from build123d import *

# Parameters (mm, degrees)
BOSS_EXTRUDE1_DEPTH      = 1
BOSS_EXTRUDE1_DEPTH_BACK = 1
SKETCH2_R                = 30
SKETCH1_R                = 9.350852961
BOSS_EXTRUDE2_DEPTH      = 14
BOSS_EXTRUDE3_DEPTH      = 15
CIRPATTERN1_COUNT        = 3
CUT_EXTRUDE2_DEPTH       = 64.041803276
SKETCH4_R                = 1
CUT_EXTRUDE3_DEPTH       = 43
CIRPATTERN2_COUNT        = 3
CUT_EXTRUDE4_DEPTH       = 43
FILLET1_R                = 10


with BuildPart() as part:
    # Sketch2 → Boss-Extrude1 (new, two sides: drawn at the far end of the back side and taken through both)
    with BuildSketch(Plane(origin=(0, 0, 0), x_dir=(1, 0, 0), z_dir=(0, 1, 0)).offset(-BOSS_EXTRUDE1_DEPTH_BACK)):
        with Locations(Location((0, 0, 0), (0, 0, 270))):
            Circle(SKETCH2_R)
    extrude(amount=BOSS_EXTRUDE1_DEPTH + BOSS_EXTRUDE1_DEPTH_BACK)

    # Sketch1 → Boss-Extrude2 (add)
    with BuildSketch(Plane(origin=(0, 1, 0), x_dir=(1, 0, 0), z_dir=(0, 1, 0))):
        with Locations(Location((0, 0, 0), (0, 0, 90))):
            Circle(SKETCH1_R)
        Polygon((3.175426481, -5.5), (6.350852961, 0), (3.175426481, 5.5), (-3.175426481, 5.5), (-6.350852961, 0), (-3.175426481, -5.5), align=None, mode=Mode.SUBTRACT)
    extrude(amount=BOSS_EXTRUDE2_DEPTH)

    # Sketch1<3> → Boss-Extrude3 (add)
    with BuildSketch(Plane(origin=(0, 1, 0), x_dir=(1, 0, 0), z_dir=(0, 1, 0))):
        with BuildLine():
            Line((2.998219694, 26.806931157), (8.371578903, 17.5))
            Line((8.371578903, 17.5), (3.315841392, 8.74320576))
            ThreePointArc((3.315841392, 8.74320576), (4.675426481, 8.098076211), (5.913917603, 7.24320576))
            Line((5.913917603, 7.24320576), (10.969655115, 16))
            Line((10.969655115, 16), (21.716373532, 16))
            Line((21.716373532, 16), (21.716373532, 19))
            Line((21.716373532, 19), (10.969655115, 19))
            Line((10.969655115, 19), (5.596295906, 28.306931157))
            Line((5.596295906, 28.306931157), (2.998219694, 26.806931157))
        make_face()
    boss_extrude3 = extrude(amount=BOSS_EXTRUDE3_DEPTH)

    # CirPattern1: Boss-Extrude3 ×3 about axis
    cirpattern1_axis = Axis((0, 0, 0), (0, 1, 0))
    for i in range(1, CIRPATTERN1_COUNT):
        add(boss_extrude3.rotate(cirpattern1_axis, i * 360 / CIRPATTERN1_COUNT))

    # Sketch3 → Cut-Extrude2 (cut, symmetric)
    with BuildSketch(Plane(origin=(-16.454482672, 0, 9.5), x_dir=(0.5000000000000041, 0, 0.8660254037844364), z_dir=(-0.8660254037844363, 0, 0.500000000000004))):
        Polygon((-19.969655115, 2.372421116), (-21.716373532, 4.828660441), (-21.716373532, 2.372421116), align=None)
        with BuildLine():
            Line((-21.716373532, 16), (-21.716373532, 15.684973294))
            ThreePointArc((-21.716373532, 15.684973294), (-20.857104699, 15.920613096), (-19.969655115, 16))
            Line((-19.969655115, 16), (-21.716373532, 16))
        make_face()
    cut_extrude2 = extrude(amount=CUT_EXTRUDE2_DEPTH, both=True, mode=Mode.SUBTRACT)

    # Sketch4 → Cut-Extrude3 (cut)
    with BuildSketch(Plane(origin=(-16.454482672, 0, 9.5), x_dir=(0.500000000000004, 0, 0.8660254037844364), z_dir=(-0.8660254037844365, 0, 0.500000000000004))):
        with Locations((-19.969655115, 11)):
            Circle(SKETCH4_R)
    cut_extrude3 = extrude(amount=-CUT_EXTRUDE3_DEPTH, mode=Mode.SUBTRACT)

    # CirPattern2: Cut-Extrude2, Cut-Extrude3 ×3 about axis
    cirpattern2_axis = Axis((0, 1, 0), (0, 1, 0))
    add([cut_extrude2.rotate(cirpattern2_axis, i * 360 / CIRPATTERN2_COUNT) for i in range(1, CIRPATTERN2_COUNT)], mode=Mode.SUBTRACT)
    add([cut_extrude3.rotate(cirpattern2_axis, i * 360 / CIRPATTERN2_COUNT) for i in range(1, CIRPATTERN2_COUNT)], mode=Mode.SUBTRACT)

    # Sketch5 → Cut-Revolve2 (revolve, cut)
    with BuildSketch(Plane(origin=(0, 0, 0), x_dir=(0, 0, -1), z_dir=(1, 0, 0)), mode=Mode.PRIVATE) as cut_revolve2_sk:
        Polygon((-26.777856991, 4), (-31.777856991, 9), (-31.777856991, -1), (-26.777856991, -1), align=None)
    revolve(cut_revolve2_sk.sketch.rotate(Axis((0, -1000, 0), (0, 1, 0)), 180), axis=Axis((0, -1000, 0), (0, 1, 0)), mode=Mode.SUBTRACT)

    # Sketch1<4> → Cut-Extrude4 (cut)
    with BuildSketch(Plane(origin=(0, 1, 0), x_dir=(1, 0, 0), z_dir=(0, 1, 0))):
        Polygon((-3.175426481, -5.5), (3.175426481, -5.5), (6.350852961, 0), (3.175426481, 5.5), (-3.175426481, 5.5), (-6.350852961, 0), align=None)
    extrude(amount=-CUT_EXTRUDE4_DEPTH, mode=Mode.SUBTRACT)

    # Fillet1
    # the kernel refuses this fillet: 10 mm, written as the material it takes off along each edge
    with BuildSketch(Plane(origin=(0, 16, 0), x_dir=(0.9612469799967569, 0, -0.27568867123462737), z_dir=(-0.27568867123462737, 0, -0.9612469799967569))) as fillet1_piece_1:
        with BuildLine():
            CenterArc((13.709751905, 10), FILLET1_R, 244.158067237, 25.841932763)
            Line((9.350852961, 1), (9.263674982, 0.82))
            ThreePointArc((9.263674982, 0.82), (9.150852961, 0.5), (9.150852961, 0))
            Line((9.150852961, 0), (9.350852961, -0.2))
            Line((9.350852961, -0.2), (13.709751905, -0.2))
            Line((13.709751905, -0.2), (13.709751905, 0))
        make_face()
    revolve(axis=Axis((0, 16, 0), (0, -1, 0)), revolution_arc=152.006117334, mode=Mode.SUBTRACT)
    with BuildSketch(Plane(origin=(0, 16, 0), x_dir=(-0.24187009717361344, 0, 0.9703086396055776), z_dir=(0.9703086396055776, 0, 0.24187009717361344))) as fillet1_piece_2:
        with BuildLine():
            CenterArc((13.709751905, 10), FILLET1_R, 244.158067237, 25.841932763)
            Line((9.350852961, 1), (9.263674982, 0.82))
            ThreePointArc((9.263674982, 0.82), (9.150852961, 0.5), (9.150852961, 0))
            Line((9.150852961, 0), (9.350852961, -0.2))
            Line((9.350852961, -0.2), (13.709751905, -0.2))
            Line((13.709751905, -0.2), (13.709751905, 0))
        make_face()
    revolve(axis=Axis((0, 16, 0), (0, -1, 0)), revolution_arc=152.006117334, mode=Mode.SUBTRACT)
    with BuildSketch(Plane(origin=(0, 16, 0), x_dir=(-0.7193768828231427, 0, -0.6946199683709492), z_dir=(-0.6946199683709492, 0, 0.7193768828231427))) as fillet1_piece_3:
        with BuildLine():
            CenterArc((13.709751905, 10), FILLET1_R, 244.158067237, 25.841932763)
            Line((13.709751905, 0), (13.709751905, -0.2))
            Line((13.709751905, -0.2), (9.350852961, -0.2))
            Line((9.350852961, -0.2), (9.150852961, 0))
            ThreePointArc((9.150852961, 0), (9.150852961, 0.5), (9.263674982, 0.82))
            Line((9.263674982, 0.82), (9.350852961, 1))
        make_face()
    revolve(axis=Axis((0, 16, 0), (0, -1, 0)), revolution_arc=152.006117334, mode=Mode.SUBTRACT)


solid = part.part
Verification items for the finished model (mm, model axes). A direction names the side the tool comes from. Give positions to 0.01 mm unless a question says otherwise; leave off trailing zeros. Order: outer loops, then holes, each group sorted by start corner. A loop starts at its lowest first (then second) coordinate and runs counter-clockwise, first axis right, second up. Notation, with made-up numbers: M -6,40.5 L 29,40.5 A31 cw 29,65.5 Z; hole C 36,28.5 d4. An arc over 180 degrees is marked long. Use one line per item in the form item = value. Start each with the question number.
Q1. Access from +Z, -Z, +X, -X, +Y, -Y to the whole of each face (thin tool, end or side, straight path). Record for faces 5 (the flat face through (-4.3, 15, -4)), 6 (the flat face through (4.74, 7.11, 2.79)), 7 (the cylindrical face through (4.7, 15.92, -26.81)), 8 (the cylindrical face through (20.87, 15.92, -17.52)), 9 (the flat face through (5.72, 8.4, 22.09)).
Q2. Section check A-A (x = 0). Enter the section's corners in (y, z), then the cut area to 3 significant figures.
Q3. Go/stop test with flat-tipped pins: pin 1 Ø8.5 at (x, y) = (16.5, 8) entering from -Z; pin 2 Ø6 at (x, y) = (-10.5, 1.5) entering from -Z; pin 3 Ø0.5 at (x, z) = (-24.5, -10) entering from +Y; pin 4 Ø1.8 at (x, y) = (19.97, 11) entering from +Z. Record where each tip stops, or that it passes through.
Q4. Section check D-D (y = 11). Count the separate pieces of the cut face and the enclosed holes in it, then the cut area to 3 significant figures.
Q5. Section check C-C (z = -4.5). Enter the section's corners in (x, y).
Q6. Scan lines: line 1 along Z through (x, y) = (19, 12); line 2 along Z through (x, y) = (-0.5, 1.25); line 3 along Z through (x, y) = (-12, 4.75). Record each from-to range of solid material in increasing order. Write a range as [from, to].
Q7. Mould release check, pull along Z, two halves, no side actions. Record for faces 1 (the flat face through (-4.785, 7.112, 2.712)), 2 (the flat face through (-21.99, 8.4, -6.09)), 3 (the conical face through (-26.06, 4.82, 9.08)), 4 (the flat face through (-4.74, 7.11, -2.79)): +Z half, -Z half, draft (parallel to the pull), parting line (faces both ways), or undercut.
Evaluation:
q1.face_5 = +Y
q1.face_6 = +Y, -Y
q1.face_7 = -Z, -X, +Y
q1.face_8 = +Z, -Z, +X, +Y
q1.face_9 = -X, +Y
q2.outline = M -1,-26.78 L 1,-26.78 L 1,-9.35 L 15,-9.35 L 15,-5.5 L -1,-5.5 Z; M -1,5.5 L 15,5.5 L 15,9.35 L 1,9.35 L 1,26.78 L -1,26.78 Z
q2.area = 193 mm2
q3.pin_1 = -19
q3.pin_2 = -25.69
q3.pin_3 = 15.95
q3.pin_4 = through
q4.separate_pieces = 7
q4.enclosed_holes = 1
q4.area = 429 mm2
q5.outline = M -26.4,-1 L -3.75,-1 L -3.75,15 L -8.2,15 L -8.2,1 L -21.07,1 L -21.07,16 L -24.54,16 L -24.54,1 L -26.4,1 Z; M 3.75,-1 L 26.4,-1 L 26.4,1 L 8.2,1 L 8.2,15 L 3.75,15 Z
q6.line_1 = [-19, -16], [16, 19]
q6.line_2 = [-9.34, -5.5], [5.5, 9.34]
q6.line_3 = [-1.5, 1.5]
q7.face_1 = undercut
q7.face_2 = -Z half
q7.face_3 = +Z half
q7.face_4 = undercut
